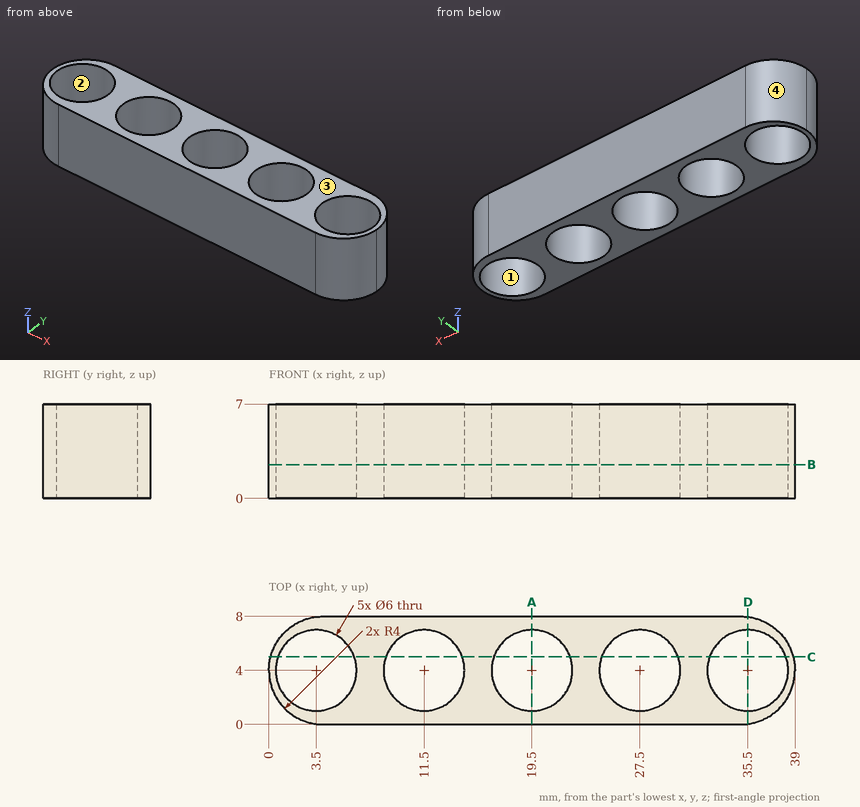
Design review of the part shown in the three views and the two pictorial views. Dimensions are in mm from the part's minimum x, y and z. Round coordinates to 2 decimals unless told otherwise and drop trailing zeros. Write each loop counter-clockwise with the first axis right and the second up, starting at its lowest first coordinate (ties: lowest second). Pieces come first, ordered by that corner, then holes. Notation, with made-up numbers: (-11.75, 22.5) - (45.25, 22.5) arc R26 cw to (45.25, 39.5) - close; hole circle Ø5 at (-11.5, 87.25). An arc over 180 degrees is marked (long way). Answer as CSV lines item,"result". Start each with the question number.
(1) Add section A-A, the plane x = 19.5. State the section outline as (y, z) points.
(2) Add section D-D, the plane x = 35.5. State the section outline as (y, z) points, plus the area to 3 significant figures.
(3) Add section B-B, the plane z = 2.5. State how many separate pieces and enclosed holes the cut face has, plus the area to 3 significant figures.
(4) For pin 1 (3 mm diameter, centred on y = 4.5, z = 4, fed in from +X), flat-tipped, find the tip position at first contact; note if it passes through.
(5) Add section C-C, the plane y = 5. State the section outline as (x, z) points, plus the area to 3 significant figures.
(6) For line 1 (Y direction, x = 19.5, z = 5); line 2 (X direction, y = 6.25, z = 2.5); line 3 (X direction, y = 6, z = 6.25), list the stretches that pass through material, from the lowest coordinate up.
(7) Mouldability with a two-part tool opening along Y and no side actions: class the marked faces 1, 2, 3 and 4 as +Y half, -Y half, draft (parallel to the pull), parting line (faces both ways), or undercut.
From the geometry:
1,outline,"(0, 0) - (1, 0) - (1, 7) - (0, 7) - close; (7, 0) - (8, 0) - (8, 7) - (7, 7) - close"
2,outline,"(0.03, 0) - (1, 0) - (1, 7) - (0.03, 7) - close; (7, 0) - (7.97, 0) - (7.97, 7) - (7, 7) - close"
2,area,"13.6 mm²"
3,separate pieces,"1"
3,enclosed holes,"5"
3,area,"157 mm²"
4,pin 1,"stops at x = 39"
5,outline,"(0.13, 0) - (0.67, 0) - (0.67, 7) - (0.13, 7) - close; (6.33, 0) - (8.67, 0) - (8.67, 7) - (6.33, 7) - close; (14.33, 0) - (16.67, 0) - (16.67, 7) - (14.33, 7) - close; (22.33, 0) - (24.67, 0) - (24.67, 7) - (22.33, 7) - close; (30.33, 0) - (32.67, 0) - (32.67, 7) - (30.33, 7) - close; (38.33, 0) - (38.87, 0) - (38.87, 7) - (38.33, 7) - close"
5,area,"73.2 mm²"
6,line 1,"y = 0 to 1, 7 to 8"
6,line 2,"x = 0.69 to 1.52, 5.48 to 9.52, 13.48 to 17.52, 21.48 to 25.52, 29.48 to 33.52, 37.48 to 38.31"
6,line 3,"x = 0.54 to 1.26, 5.74 to 9.26, 13.74 to 17.26, 21.74 to 25.26, 29.74 to 33.26, 37.74 to 38.46"
7,face 1,"undercut"
7,face 2,"undercut"
7,face 3,"draft"
7,face 4,"+Y half"
